```python
from build123d import *

# Parameters (mm, degrees)
SKETCH1_R               = 25.736334191
BOSS_EXTRUDE1_DEPTH     = 0.1
CUT_EXTRUDE1_DEPTH      = 147.870107232
CUT_EXTRUDE1_DEPTH_BACK = 147.870107232
SKETCH2_R               = 10


with BuildPart() as part:
    # Sketch1 → Boss-Extrude1 (new body)
    with BuildSketch(Plane(origin=(0, 0, 0), x_dir=(1, 0, 0), z_dir=(0, 1, 0))):
        with BuildLine():
            Line((-76.705846626, 6.628303893), (-76.705846626, -41.491355388))
            ThreePointArc((-76.705846626, -41.491355388), (-75.563563073, -44.249071834), (-72.805846626, -45.391355388))
            Line((-72.805846626, -45.391355388), (135.779788281, -45.391355388))
            ThreePointArc((135.779788281, -45.391355388), (138.537504728, -44.249071834), (139.679788281, -41.491355388))
            Line((139.679788281, -41.491355388), (139.679788281, 6.628303893))
            ThreePointArc((139.679788281, 6.628303893), (138.537504728, 9.386020339), (135.779788281, 10.528303893))
            Line((135.779788281, 10.528303893), (-72.805846626, 10.528303893))
            ThreePointArc((-72.805846626, 10.528303893), (-75.563563073, 9.386020339), (-76.705846626, 6.628303893))
        make_face()
        with Locations(Location((-43.538029172, -17.431525748, 0), (0, 0, 270))):
            Circle(SKETCH1_R, mode=Mode.SUBTRACT)
    extrude(amount=BOSS_EXTRUDE1_DEPTH)

    # Sketch2 → Cut-Extrude1 (cut, two sides: drawn at the far end of the back side and taken through both)
    with BuildSketch(Plane(origin=(0, 0.1, 0), x_dir=(1, 0, 0), z_dir=(0, 1, 0)).offset(-CUT_EXTRUDE1_DEPTH_BACK)):
        with Locations(Location((11.461970828, -17.431525748, 0), (0, 0, 270))):
            Circle(SKETCH2_R)
        with Locations(Location((46.461970828, -17.431525748, 0), (0, 0, 270))):
            Circle(SKETCH2_R)
        with Locations(Location((81.461970828, -17.431525748, 0), (0, 0, 270))):
            Circle(SKETCH2_R)
        with Locations(Location((116.461970828, -17.431525748, 0), (0, 0, 270))):
            Circle(SKETCH2_R)
    extrude(amount=CUT_EXTRUDE1_DEPTH + CUT_EXTRUDE1_DEPTH_BACK, mode=Mode.SUBTRACT)


solid = part.part
```
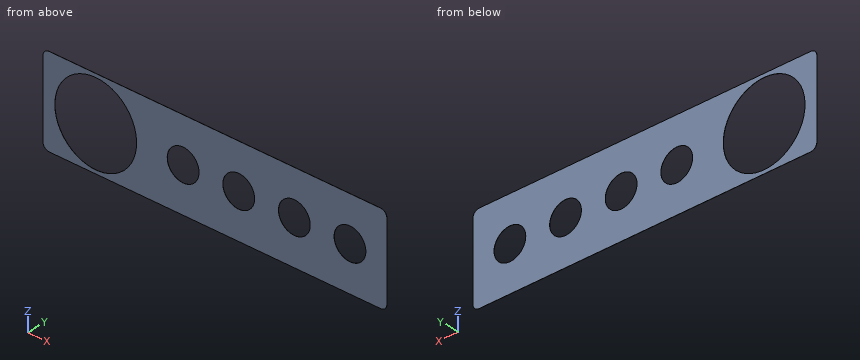
Work out the finished part from the listing and answer in its coordinate system (mm). Give positions to 0.01 mm unless a question says otherwise; leave off trailing zeros. Write each loop counter-clockwise with the first axis right and the second up, starting at its lowest first coordinate (ties: lowest second). Pieces come first, ordered by that corner, then holes. Notation, with made-up numbers: (-33.75, 40.5) - (-20.75, 40.5) arc R22 cw to (-20.75, 68.5) - close; hole circle Ø3 at (74, -18.5). An arc over 180 degrees is marked (long way). Use one line per item in the form item = value.
1. A cutting plane is placed at D-D (z = -1). Write down the section's boundary in (x, y), and give its area (3 significant figures).
Filled in:
outline = (-76.71, 0) - (-61.5, 0) - (-61.5, 0.1) - (-76.71, 0.1) - close; (-25.58, 0) - (139.68, 0) - (139.68, 0.1) - (-25.58, 0.1) - close
area = 18.0 mm^2
2. A cutting plane is placed at C-C (y = 0.05). Write down the section's boundary in (x, z), and give its area (3 significant figures).
Filled in:
outline = (-76.71, -6.63) arc R3.9 ccw to (-72.81, -10.53) - (135.78, -10.53) arc R3.9 ccw to (139.68, -6.63) - (139.68, 41.49) arc R3.9 ccw to (135.78, 45.39) - (-72.81, 45.39) arc R3.9 ccw to (-76.71, 41.49) - close; hole circle Ø51.47 at (-43.54, 17.43); hole circle Ø20 at (11.46, 17.43); hole circle Ø20 at (46.46, 17.43); hole circle Ø20 at (81.46, 17.43); hole circle Ø20 at (116.46, 17.43)
area = 8,750 mm^2
3. A cutting plane is placed at B-B (z = 19.5). Write down the section's boundary in (x, y).
Filled in:
outline = (-76.71, 0) - (-69.19, 0) - (-69.19, 0.1) - (-76.71, 0.1) - close; (-17.88, 0) - (1.68, 0) - (1.68, 0.1) - (-17.88, 0.1) - close; (21.25, 0) - (36.68, 0) - (36.68, 0.1) - (21.25, 0.1) - close; (56.25, 0) - (71.68, 0) - (71.68, 0.1) - (56.25, 0.1) - close; (91.25, 0) - (106.68, 0) - (106.68, 0.1) - (91.25, 0.1) - close; (126.25, 0) - (139.68, 0) - (139.68, 0.1) - (126.25, 0.1) - close
4. Consider L1, parallel to X at y = 0.05, z = 12; L2, parallel to Z at x = 113.5, y = 0.05; L3, parallel to X at y = 0.05, z = 31. Determine where each line is inside the solid, lowest interval first.
Filled in:
L1 = -76.71 to -68.69, -18.38 to 3.07, 19.86 to 38.07, 54.86 to 73.07, 89.86 to 108.07, 124.86 to 139.68
L2 = -10.53 to 7.88, 26.98 to 45.39
L3 = -76.71 to -65.41, -21.67 to 139.68
5. A cutting plane is placed at A-A (z = 30). Write down the section's boundary in (x, y).
Filled in:
outline = (-76.71, 0) - (-66, 0) - (-66, 0.1) - (-76.71, 0.1) - close; (-21.08, 0) - (139.68, 0) - (139.68, 0.1) - (-21.08, 0.1) - close
